Answer from the drawing. Dimensions are ordinates in mm from the lowest x, y and z of the part. Coordinates: 2 decimals unless noted, no trailing zeros. Loops run counter-clockwise (first coordinate to the right, second up) from the corner with the lowest first, then second, coordinate; pieces in that order, holes last. Notation, with made-up numbers: (15.5, 24) - (64.5, 24) arc R20 ccw to (64.5, 40) - close; hole circle Ø4 at (71, 6.5). An arc over 180 degrees is marked (long way). One line per question, with ' | ' between items. Start each with the question number.
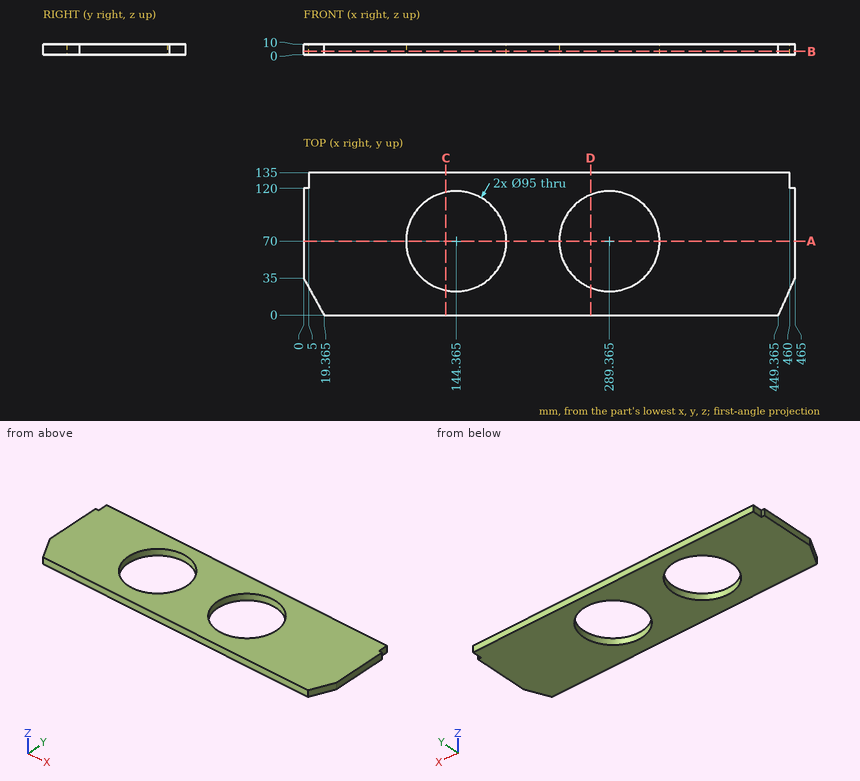
1) The part is cut by section A-A on y = 70. Write down the section's boundary in (x, z) (3 decimals), and give its area (3 significant figures).
2) Find the intervals of material crossed by line 1 along X through (y, z) = (42, 7.25) (1 decimal); line 2 along X through (y, z) = (57, 0.75); line 3 along Y through (x, z) = (108, 1.75), in increasing order. Write a range as from..to.
3) The part is cut by section B-B on z = 3. Write down the section's boundary in (x, y) (3 decimals), and give its area (3 significant figures).
4) Given pin 1 Ø1.5 at (x, y) = (220, 19) entering from -Z; pin 2 Ø3 at (y, z) = (130.5, 6.5) entering from -X; pin 3 Ø3 at (y, z) = (16.5, 3) entering from -X; pin 4 Ø1.5 at (x, z) = (463, 3) entering from +Y, each flat-ended and moving along its own axis, determine where each tip first touches the part or whether it passes through.
5) The part is cut by section C-C on x = 134.5. Write down the section's boundary in (y, z).
6) The part is cut by section D-D on x = 271.5. Write down the section's boundary in (y, z), and give its area (3 significant figures).
Answer below:
1) outline: (0, 0) - (96.865, 0) - (96.865, 10) - (0, 10) - close; (191.865, 0) - (241.865, 0) - (241.865, 10) - (191.865, 10) - close; (336.865, 0) - (465, 0) - (465, 10) - (336.865, 10) - close | area: 2,750 mm2
2) line 1: 0..106, 182.7..251, 327.7..465 | line 2: 0..98.68, 190.05..243.68, 335.05..465 | line 3: 0..39.44, 100.56..135
3) outline: (0, 35) - (19.365, 0) - (449.365, 0) - (465, 35) - (465, 120) - (460, 120) - (460, 135) - (5, 135) - (5, 120) - (0, 120) - close; hole circle Ø95 at (144.365, 70); hole circle Ø95 at (289.365, 70) | area: 47,800 mm2
4) pin 1: z = 0 | pin 2: x = 5 | pin 3: x = 9.41 | pin 4: y = 120
5) outline: (0, 0) - (23.54, 0) - (23.54, 10) - (0, 10) - close; (116.46, 0) - (135, 0) - (135, 10) - (116.46, 10) - close
6) outline: (0, 0) - (25.99, 0) - (25.99, 10) - (0, 10) - close; (114.01, 0) - (135, 0) - (135, 10) - (114.01, 10) - close | area: 470 mm2
